```python
from build123d import *

# Parameters (mm, degrees)
BOSS_EXTRUDE1_DEPTH     = 2
SKETCH9_R               = 4.76
CUT_EXTRUDE1_DEPTH      = 15
CUT_EXTRUDE1_DEPTH_BACK = 16


with BuildPart() as part:
    # Sketch2 → Boss-Extrude1 (new body)
    with BuildSketch(Plane.XY):
        with BuildLine():
            Line((-10, -3.679637035), (-10, 13.820362965))
            ThreePointArc((-10, 13.820362965), (-7.492138287, 58.541722515), (0, 102.702307138))
            ThreePointArc((0, 102.702307138), (7.492138287, 58.541722515), (10, 13.820362965))
            Line((10, 13.820362965), (10, -3.679637035))
            ThreePointArc((10, -3.679637035), (7.492466261, -48.398081393), (0.001303671, -92.555860711))
            Line((0.001303671, -92.555860711), (-0.001303671, -92.555860711))
            ThreePointArc((-0.001303671, -92.555860711), (-7.492466261, -48.398081393), (-10, -3.679637035))
        make_face()
    extrude(amount=BOSS_EXTRUDE1_DEPTH)

    # Sketch9 → Cut-Extrude1 (cut, two sides)
    with BuildSketch(Plane(origin=(0, 0, 0), x_dir=(-1, 0, 0), z_dir=(0, 0, -1))) as cut_extrude1_sk:
        with Locations((-0.000651835, 5.073223214)):
            Circle(SKETCH9_R)
    extrude(amount=CUT_EXTRUDE1_DEPTH, mode=Mode.SUBTRACT)
    extrude(cut_extrude1_sk.sketch, amount=-CUT_EXTRUDE1_DEPTH_BACK, mode=Mode.SUBTRACT)


solid = part.part
```
The listing builds one solid part. Answer for the finished solid, in the listing's coordinates (mm). Round coordinates to 2 decimals unless told otherwise and drop trailing zeros. Loops run counter-clockwise (first coordinate to the right, second up) from the corner with the lowest first, then second, coordinate; pieces in that order, holes last. Notation, with made-up numbers: (56, -8) - (108, -8) arc R25 cw to (108, 22) - close; hole circle Ø3 at (17, 15). An arc over 180 degrees is marked (long way). Use one line per item in the form item = value. Start each with the question number.
1. The part is cut by section C-C on y = -63.5. Determine the outline of the cut face in (x, z), then the cut area to 3 significant figures.
2. The part is cut by section A-A on x = -2.75. Determine the outline of the cut face in (y, z).
3. Consider line 1 (X direction, y = 17, z = 0.75); line 2 (X direction, y = -70, z = 1.8). Determine where each line is inside the solid, lowest interval first. Write a range as [from, to].
4. For a pull along X with two mould halves and no side action, classify faces 1 (the face through (7.42, 59.17, 0.99)), 2 (the face through (1.033, 0.426, 0.986)), 3 (the face through (5, 6, 2)), 4 (the face through (-7.42, -49.02, 0.99)) as pulls with the +X half, pulls with the -X half, needs draft (parallel to the pull), parting line crosses it, or undercut.
Geometry check:
q1.outline = (-5.5, 0) - (5.5, 0) - (5.5, 2) - (-5.5, 2) - close
q1.area = 22.0 mm^2
q2.outline = (-79.49, 0) - (1.19, 0) - (1.19, 2) - (-79.49, 2) - close; (8.96, 0) - (89.63, 0) - (89.63, 2) - (8.96, 2) - close
q3.line_1 = [-9.99, 9.99]
q3.line_2 = [-4.46, 4.46]
q4.face_1 = pulls with the +X half
q4.face_2 = undercut
q4.face_3 = needs draft
q4.face_4 = pulls with the -X half
